The drawing under review shows one solid part. Ordinate dimensions are in mm from its lowest x, y, z. Give positions to 0.01 mm unless a question says otherwise; leave off trailing zeros. Write each loop counter-clockwise with the first axis right and the second up, starting at its lowest first coordinate (ties: lowest second). Pieces come first, ordered by that corner, then holes. Notation, with made-up numbers: M -7,41 L 32,41 A18 ccw 32,51 Z; hole C 65,1.5 d2. An arc over 180 degrees is marked long. Answer as a JSON object with one key per item and string values. Group by question number.
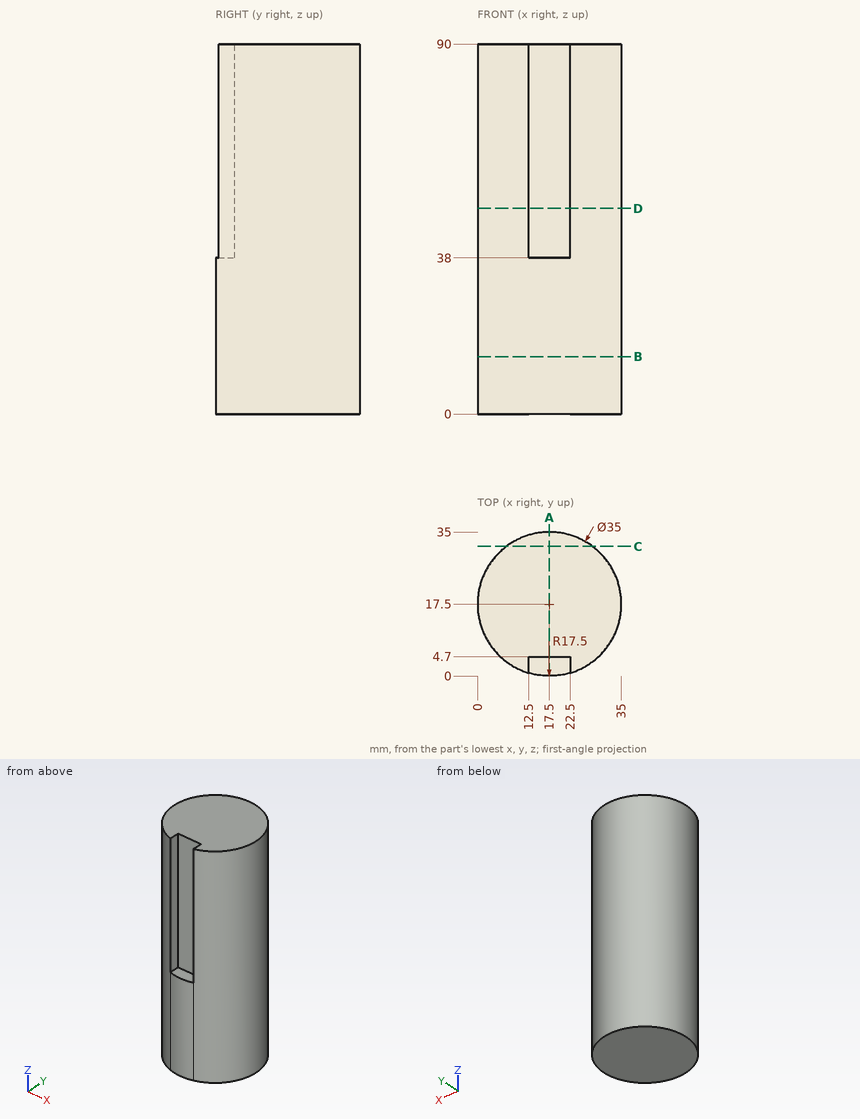
Item 1: Insertion check: P1, Ø1.5, axis at x = 19, z = 77, coming from the -Y side; P2, Ø4, axis at y = 22.5, z = 68, coming from the -X side; P3, Ø4.5, axis at y = 2, z = 52.5, coming from the +X side. Each pin has a flat end and moves straight along its axis. Give the tip position at first contact, or say it passes through.
Item 2: Consider section B-B (z = 14). Give the boundary of the cut face in (x, y).
Item 3: Consider section D-D (z = 50). Give the boundary of the cut face in (x, y).
Item 4: Consider section A-A (x = 17.5). Give the boundary of the cut face in (y, z).
Item 5: Consider section C-C (y = 31.5). Give the boundary of the cut face in (x, z), plus the area to 3 significant figures.
Item 6: To check wall thickness, follow probe 1 along Z at (x, y) = (15.5, 2.5); probe 2 along X at (y, z) = (18, 12); probe 3 along X at (y, z) = (3, 51.5). State the ranges of each line that lie inside material, in increasing order.
Result set:
{
 "1": {"P1": "stops at y = 4.7", "P2": "stops at x = 0.26", "P3": "stops at x = 28.93"},
 "2": {"outline": "C 17.5,17.5 d35"},
 "3": {"outline": "M 12.5,0.73 L 12.5,4.7 L 22.5,4.7 L 22.5,0.73 A17.5 ccw long Z"},
 "4": {"outline": "M 0,0 L 35,0 L 35,90 L 4.7,90 L 4.7,38 L 0,38 Z"},
 "5": {"outline": "M 7,0 L 28,0 L 28,90 L 7,90 Z", "area": "1,890 mm^2"},
 "6": {"probe 1": "z = 0 to 38", "probe 2": "x = 0.01 to 34.99", "probe 3": "x = 7.7 to 12.5, 22.5 to 27.3"}
}
